Geometry check sheet. Reference: the model listing, model coordinates, mm. Face numbers are marked on the shaded views. A direction names the side the tool comes from. Coordinates: 2 decimals unless noted, no trailing zeros. Loops run counter-clockwise (first coordinate to the right, second up) from the corner with the lowest first, then second, coordinate; pieces in that order, holes last. Notation, with made-up numbers: (-38.5, -37.75) - (9.5, -37.75) arc R21 ccw to (9.5, -31.75) - close; hole circle Ø2 at (77.5, 32). An arc over 180 degrees is marked (long way). Write each question's results on one line, items separated by ' | '. Start each with the question number.
(1) Sectioned sample at C-C (x = -2.15). Enter the section's corners in (y, z), plus the area to 3 significant figures.
(2) Sectioned sample at B-B (z = 3). Enter the section's corners in (x, y).
(3) Go/stop test with flat-tipped pins: pin 1 Ø9.5 at (y, z) = (0, 0) entering from +X; pin 2 Ø0.7 at (x, z) = (-5, -2) entering from +Y; pin 3 Ø1 at (x, y) = (-2.5, 6) entering from -Z. Record where each tip stops, or that it passes through.
(4) Material ranges on probe 1 along Y at (x, z) = (-3.4, 0); probe 2 along Y at (x, z) = (-0.7, 0); probe 3 along X at (y, z) = (-9.5, -4.25), recorded low to high.
(5) Sectioned sample at A-A (y = 0). Enter the section's corners in (x, z).
(6) Mould release check, pull along Y, two halves, no side actions. Record for the marked faces 4, 5 and 6: pulls with the +Y half, pulls with the -Y half, needs draft (parallel to the pull), parting line crosses it, or undercut.
(7) Sectioned sample at D-D (y = -7.25). Enter the section's corners in (x, z).
(8) Access from +Z, -Z, +X, -X, +Y, -Y to the whole of each face (thin tool, end or side, straight path). Record for the marked faces 1, 2 and 3.
from build123d import *

# Parameters (mm, degrees)
SKETCH1_W          = 5
SKETCH1_H          = 6.4
SKETCH2_W          = 3
SKETCH2_H          = 1.5
SKETCH3_R          = 7.9
CUT_EXTRUDE1_DEPTH = 0.8
CUT_EXTRUDE2_DEPTH = 1


with BuildPart() as part:
    # Sketch1 → Revolve1 (revolve)
    with BuildSketch(Plane.XY, mode=Mode.PRIVATE) as revolve1_sk:
        with Locations((-3, 7.3)):
            Rectangle(SKETCH1_W, SKETCH1_H)
    revolve(revolve1_sk.sketch.rotate(Axis((0, 0, 0), (1, 0, 0)), 90), axis=Axis((0, 0, 0), (1, 0, 0)))

    # Sketch2 → Cut-Revolve1 (revolve, cut)
    with BuildSketch(Plane.XY, mode=Mode.PRIVATE) as cut_revolve1_sk:
        with Locations((-3, 9.75)):
            Rectangle(SKETCH2_W, SKETCH2_H)
    revolve(cut_revolve1_sk.sketch.rotate(Axis((0, 0, 0), (1, 0, 0)), 90), axis=Axis((0, 0, 0), (1, 0, 0)), mode=Mode.SUBTRACT)

    # Sketch3 → Cut-Extrude1 (cut)
    with BuildSketch(Plane(origin=(0, 0, 0), x_dir=(0, 0, -1), z_dir=(1, 0, 0))):
        Circle(SKETCH3_R)
    extrude(amount=-CUT_EXTRUDE1_DEPTH, mode=Mode.SUBTRACT)

    # Sketch5 → Cut-Extrude2 (cut)
    # profile 1 of 2: a face of its own
    with BuildSketch(Plane.ZY.offset(5.5)):
        Polygon((-1.793384415, 7.675), (-0.9125, 7.675), (-0.9125, 4.5), (-1.482371795, 4.5), (-1.482371795, 7.145833333), (-2.133653846, 7.145833333), align=None)
    # profile 2 of 2: a face of its own
    with BuildSketch(Plane.ZY.offset(5.5)):
        with BuildLine():
            add(Edge.make_bspline(
                [(1.786758814, 6.209615385), (1.820052688, 6.185826012), (1.885954908, 6.138737096), (1.972987633, 6.054375541), (2.047953153, 5.960269248), (2.110064245, 5.856995446), (2.159825779, 5.747092633), (2.195447488, 5.631735537), (2.218073988, 5.511941637), (2.220545477, 5.430382608), (2.221794872, 5.389152644)],
                knots=[0, 0, 0, 0, 1.013736912, 2.006600758, 2.994453809, 3.989973287, 4.987781207, 5.978959008, 6.978317308, 8, 8, 8, 8], degree=3))
            add(Edge.make_bspline(
                [(2.221794872, 5.389152644), (2.220287572, 5.34450785), (2.217298037, 5.255960631), (2.190866551, 5.126106148), (2.14843186, 5.00135344), (2.090436575, 4.883079461), (2.017721153, 4.774959714), (1.932964566, 4.679242926), (1.836059971, 4.598428905), (1.745839049, 4.543597114), (1.668182749, 4.507173392), (1.605514797, 4.483862941), (1.539341558, 4.46334135), (1.469190831, 4.446945961), (1.395075371, 4.434146669), (1.31710095, 4.42569404), (1.235216239, 4.419549495), (1.179374328, 4.418915055), (1.150741186, 4.418589744)],
                knots=[0, 0, 0, 0, 1.313679292, 2.605514271, 3.884962679, 5.186178731, 6.472827995, 7.711026938, 8.938935107, 10.174644318, 10.808706728, 11.462743532, 12.142127587, 12.847854939, 13.582806024, 14.355735269, 15.156897313, 16, 16, 16, 16], degree=3))
            add(Edge.make_bspline(
                [(1.150741186, 4.418589744), (1.120206781, 4.41900393), (1.060579108, 4.419812753), (0.973535988, 4.424703329), (0.891428611, 4.433719654), (0.814084743, 4.445588948), (0.741578798, 4.461295464), (0.673908628, 4.481210467), (0.610910835, 4.503885913), (0.533798227, 4.538411225), (0.4456725, 4.592329893), (0.350424526, 4.671292228), (0.266821174, 4.765338836), (0.194135977, 4.871829843), (0.136842765, 4.990110116), (0.094237825, 5.116467223), (0.069006675, 5.250558751), (0.065969127, 5.342404855), (0.064423077, 5.389152644)],
                knots=[0, 0, 0, 0, 0.886964665, 1.7320671, 2.531131818, 3.285397207, 4.004107883, 4.684213108, 5.332925796, 5.947568694, 7.135706876, 8.320776993, 9.52873045, 10.778999824, 12.05415135, 13.333578234, 14.642845846, 16, 16, 16, 16], degree=3))
            add(Edge.make_bspline(
                [(0.064423077, 5.389152644), (0.065835907, 5.4299324), (0.068612291, 5.510069557), (0.088499898, 5.627495836), (0.122601102, 5.738829844), (0.169393262, 5.844846641), (0.229730957, 5.945558024), (0.30397099, 6.040222955), (0.391172072, 6.129695445), (0.457298282, 6.182533521), (0.491190905, 6.209615385)],
                knots=[0, 0, 0, 0, 1.01821053, 2.000906977, 2.963938143, 3.919209931, 4.888045165, 5.887808425, 6.917407893, 8, 8, 8, 8], degree=3))
            add(Edge.make_bspline(
                [(0.491190905, 6.209615385), (0.470179277, 6.233849224), (0.428813708, 6.281558356), (0.375286255, 6.358342401), (0.33019163, 6.437506832), (0.291904146, 6.518409188), (0.263601062, 6.602442406), (0.242197406, 6.68828531), (0.230091519, 6.776812445), (0.228199332, 6.836482365), (0.22724359, 6.866621595)],
                knots=[0, 0, 0, 0, 1.061529281, 2.089831458, 3.092927091, 4.075998741, 5.048384512, 6.024008542, 7.00192825, 8, 8, 8, 8], degree=3))
            add(Edge.make_bspline(
                [(0.22724359, 6.866621595), (0.228510758, 6.907421227), (0.231010833, 6.987917329), (0.25315385, 7.105621637), (0.289916635, 7.217464189), (0.339929274, 7.323117526), (0.403437554, 7.420279049), (0.47889914, 7.507411214), (0.567374874, 7.581322406), (0.665574579, 7.64474147), (0.773990481, 7.695184406), (0.89159394, 7.730480594), (1.016964877, 7.752824943), (1.103366784, 7.755196971), (1.147561098, 7.756410256)],
                knots=[0, 0, 0, 0, 1.022455555, 2.017265428, 2.990720743, 3.968117071, 4.939886797, 5.893155559, 6.847550415, 7.820889576, 8.817530429, 9.83499769, 10.892607882, 12, 12, 12, 12], degree=3))
            add(Edge.make_bspline(
                [(1.147561098, 7.756410256), (1.191118898, 7.755194985), (1.276047488, 7.752825462), (1.399215198, 7.730629167), (1.514277223, 7.694546749), (1.620282085, 7.643038738), (1.717466215, 7.579497441), (1.804438236, 7.503012731), (1.879663021, 7.413710397), (1.94369846, 7.314035335), (1.994724865, 7.206649897), (2.032448506, 7.094033972), (2.054268305, 6.977072732), (2.057399401, 6.897661569), (2.058974359, 6.857717348)],
                knots=[0, 0, 0, 0, 1.094655142, 2.134348324, 3.136019022, 4.118575226, 5.088726318, 6.048298823, 7.020513804, 8.015920439, 9.020015034, 10.003048569, 10.995523219, 12, 12, 12, 12], degree=3))
            add(Edge.make_bspline(
                [(2.058974359, 6.857717348), (2.058215664, 6.829486932), (2.056726782, 6.774086853), (2.045718289, 6.692466901), (2.027181337, 6.614152447), (2.00133663, 6.537250953), (1.965403664, 6.459672577), (1.916778006, 6.379930777), (1.857631279, 6.294712264), (1.811180399, 6.238938489), (1.786758814, 6.209615385)],
                knots=[0, 0, 0, 0, 0.940746401, 1.846144481, 2.739104268, 3.619506754, 4.545839139, 5.581956076, 6.728711598, 8, 8, 8, 8], degree=3))
        make_face()
        with BuildLine():
            add(Edge.make_bspline(
                [(1.13356871, 7.186538462), (1.110105898, 7.185407337), (1.064465545, 7.183207049), (0.999342106, 7.163347019), (0.940794009, 7.130864527), (0.890157731, 7.086162225), (0.848633343, 7.031922679), (0.8181152, 6.969563237), (0.80001758, 6.899853484), (0.798101595, 6.851041394), (0.797115385, 6.825916466)],
                knots=[0, 0, 0, 0, 1.018099191, 1.980427864, 2.929421084, 3.909248076, 4.895556904, 5.880788387, 6.909183412, 8, 8, 8, 8], degree=3))
            add(Edge.make_bspline(
                [(0.797115385, 6.825916466), (0.798333656, 6.800576967), (0.800712448, 6.751099152), (0.819418974, 6.680050049), (0.851304765, 6.615659356), (0.89508374, 6.559271984), (0.948282285, 6.513216409), (1.007848346, 6.478041724), (1.074442524, 6.457961409), (1.120719086, 6.455238447), (1.14438101, 6.453846154)],
                knots=[0, 0, 0, 0, 1.07118507, 2.091592095, 3.082435519, 4.092579768, 5.090825648, 6.043203473, 6.999459622, 8, 8, 8, 8], degree=3))
            add(Edge.make_bspline(
                [(1.14438101, 6.453846154), (1.168490274, 6.454924942), (1.215459644, 6.457026624), (1.282220098, 6.477627967), (1.342362736, 6.510575617), (1.393866019, 6.557156306), (1.436526559, 6.613564099), (1.467595246, 6.679080076), (1.485477259, 6.752473276), (1.487864571, 6.803768386), (1.489102564, 6.83036859)],
                knots=[0, 0, 0, 0, 1.008803858, 1.965339183, 2.900766489, 3.864508618, 4.855158575, 5.849593072, 6.884859315, 8, 8, 8, 8], degree=3))
            add(Edge.make_bspline(
                [(1.489102564, 6.83036859), (1.487833255, 6.855476908), (1.485378456, 6.904035512), (1.467776605, 6.973749787), (1.435449925, 7.035135947), (1.392976839, 7.089038677), (1.339726971, 7.132507876), (1.277907775, 7.164475387), (1.207974461, 7.183016853), (1.158907715, 7.185339172), (1.13356871, 7.186538462)],
                knots=[0, 0, 0, 0, 1.065910571, 2.061433587, 3.023559535, 3.990682701, 4.956464619, 5.918590567, 6.925120432, 8, 8, 8, 8], degree=3))
        make_face(mode=Mode.SUBTRACT)
        with BuildLine():
            add(Edge.make_bspline(
                [(1.152013221, 5.883974359), (1.13418326, 5.883678266), (1.09904063, 5.88309467), (1.047378076, 5.876364936), (0.997802545, 5.866335968), (0.950375546, 5.852501289), (0.905336675, 5.833641141), (0.862304152, 5.810904884), (0.821426594, 5.784062683), (0.783310327, 5.753601858), (0.748862129, 5.720168201), (0.717810211, 5.68529798), (0.692429653, 5.648089706), (0.671293699, 5.609780194), (0.654310841, 5.570065862), (0.643083888, 5.528292696), (0.635855302, 5.485016998), (0.634818075, 5.455539347), (0.634294872, 5.440670072)],
                knots=[0, 0, 0, 0, 1.129580664, 2.226389355, 3.296443603, 4.333934503, 5.352185725, 6.386189251, 7.41493955, 8.447544828, 9.47401038, 10.455044306, 11.4018853, 12.322125673, 13.225630306, 14.132028716, 15.057747923, 16, 16, 16, 16], degree=3))
            add(Edge.make_bspline(
                [(0.634294872, 5.440670072), (0.63454424, 5.425162887), (0.63503883, 5.394406304), (0.642508927, 5.349514587), (0.653264548, 5.306219609), (0.66837116, 5.264926636), (0.688573384, 5.225659711), (0.712695206, 5.188037072), (0.741577744, 5.152322538), (0.774437858, 5.118707595), (0.81122461, 5.088380917), (0.850872666, 5.061662584), (0.892858367, 5.038106335), (0.938442094, 5.021140191), (0.985935698, 5.005611286), (1.036611549, 4.996190273), (1.089916154, 4.98925803), (1.126335289, 4.988731586), (1.145017027, 4.988461538)],
                knots=[0, 0, 0, 0, 0.973817353, 1.931446211, 2.852767904, 3.776304432, 4.688323523, 5.623710549, 6.581246645, 7.570897993, 8.57436511, 9.572506873, 10.574556662, 11.591826551, 12.624694332, 13.712108235, 14.826391851, 16, 16, 16, 16], degree=3))
            add(Edge.make_bspline(
                [(1.145017027, 4.988461538), (1.163901485, 4.988803842), (1.200701313, 4.989470882), (1.25449526, 4.995366257), (1.305374788, 5.004720502), (1.353279122, 5.018099252), (1.398389413, 5.035237963), (1.440100547, 5.057052151), (1.479364857, 5.081773696), (1.514920581, 5.110655854), (1.547385577, 5.142131378), (1.57535873, 5.176625875), (1.599143992, 5.213030128), (1.618329397, 5.251737483), (1.633810296, 5.292565228), (1.644429222, 5.335920457), (1.651018647, 5.381315958), (1.651618364, 5.412238245), (1.651923077, 5.42794972)],
                knots=[0, 0, 0, 0, 1.200705402, 2.339794563, 3.437264955, 4.487414319, 5.499029866, 6.500076882, 7.476298407, 8.444948224, 9.407950986, 10.347155707, 11.263432813, 12.167927724, 13.089546445, 14.03463663, 15.00140776, 16, 16, 16, 16], degree=3))
            add(Edge.make_bspline(
                [(1.651923077, 5.42794972), (1.651341254, 5.443866599), (1.650203992, 5.474978582), (1.643981063, 5.520922743), (1.632307482, 5.564478525), (1.617035028, 5.606656097), (1.596719157, 5.646582665), (1.571497443, 5.684173963), (1.542788942, 5.720361173), (1.509235047, 5.753533371), (1.472549081, 5.783864551), (1.433502717, 5.810886303), (1.392216224, 5.833771234), (1.348576668, 5.852478529), (1.3024246, 5.866343167), (1.254112164, 5.876364584), (1.203718609, 5.883096176), (1.169419787, 5.88367872), (1.152013221, 5.883974359)],
                knots=[0, 0, 0, 0, 1.011708178, 1.977538892, 2.938094892, 3.871441737, 4.823268678, 5.775953079, 6.743660653, 7.753304209, 8.767430709, 9.76505158, 10.765940967, 11.761741361, 12.775867861, 13.822051386, 14.89469657, 16, 16, 16, 16], degree=3))
        make_face(mode=Mode.SUBTRACT)
    extrude(amount=-CUT_EXTRUDE2_DEPTH, mode=Mode.SUBTRACT)


solid = part.part
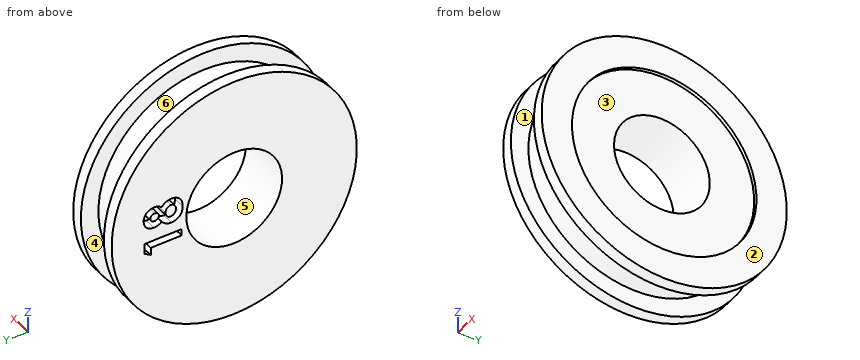
Outcome:
1) outline: circle Ø18 at (0, 0); hole circle Ø8.2 at (0, 0) | area: 202 mm2
2) outline: (-5.5, -10.06) - (-4.5, -10.06) - (-4.5, -8.49) - (-1.5, -8.49) - (-1.5, -10.06) - (-0.5, -10.06) - (-0.5, -7.31) - (-0.8, -7.31) - (-0.8, -2.79) - (-5.5, -2.79) - close; (-5.5, 2.79) - (-0.8, 2.79) - (-0.8, 7.31) - (-0.5, 7.31) - (-0.5, 10.06) - (-1.5, 10.06) - (-1.5, 8.49) - (-4.5, 8.49) - (-4.5, 10.06) - (-5.5, 10.06) - close
3) pin 1: stops at x = -0.8 | pin 2: stops at y = 10.37 | pin 3: stops at z = -7.12
4) probe 1: y = -9 to -4.1, 4.1 to 9 | probe 2: y = -10.5 to -7.9, 7.9 to 10.5 | probe 3: x = -5.5 to -4.5, -1.5 to -0.5
5) outline: (-5.5, -10.5) - (-4.5, -10.5) - (-4.5, -9) - (-1.5, -9) - (-1.5, -10.5) - (-0.5, -10.5) - (-0.5, -7.9) - (-0.8, -7.9) - (-0.8, -4.1) - (-5.5, -4.1) - close; (-5.5, 4.1) - (-0.8, 4.1) - (-0.8, 7.9) - (-0.5, 7.9) - (-0.5, 10.5) - (-1.5, 10.5) - (-1.5, 9) - (-4.5, 9) - (-4.5, 10.5) - (-5.5, 10.5) - close
6) face 4: needs draft | face 5: undercut | face 6: parting line crosses it
7) outline: (-5.5, -7.6) - (-4.5, -7.6) - (-4.5, -5.33) - (-1.5, -5.33) - (-1.5, -7.6) - (-0.5, -7.6) - (-0.5, -3.14) - (-0.8, -3.14) - (-0.8, 3.14) - (-0.5, 3.14) - (-0.5, 7.6) - (-1.5, 7.6) - (-1.5, 5.33) - (-4.5, 5.33) - (-4.5, 7.6) - (-5.5, 7.6) - close
8) face 1: none | face 2: +Z, -Z, +X, +Y, -Y | face 3: +X
